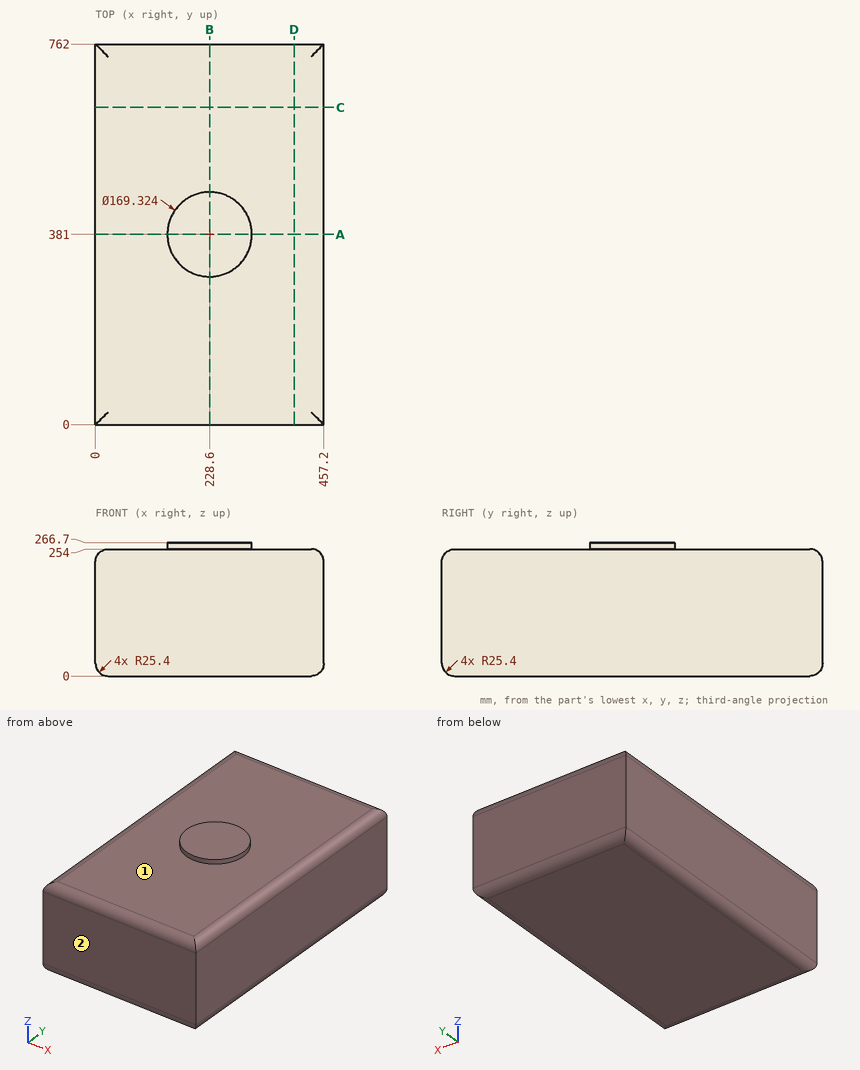
The figure shows three views and two pictorial views of one solid part (mm, origin at its lowest corner). Answer the questions. A direction names the side the tool comes from. Round coordinates to 2 decimals unless told otherwise and drop trailing zeros. Write each loop counter-clockwise with the first axis right and the second up, starting at its lowest first coordinate (ties: lowest second). Pieces come first, ordered by that corner, then holes. Notation, with made-up numbers: M -15.75,36.5 L 40.25,36.5 A37 ccw 40.25,72.5 Z; hole C 21,77 d3. An arc over 180 degrees is marked long. Write each question's results on one line, items separated by ' | '. Start each with the question number.
(1) The part is cut by section B-B, the plane x = 228.6. Write down the section's boundary in (y, z), and give its area (3 significant figures).
(2) Find the intervals of material crossed by line 1 (Z direction, x = 80, y = 39); line 2 (X direction, y = 315.5, z = 14); line 3 (X direction, y = 716, z = 235), in increasing order.
(3) This flat-tipped pin is pushed along its axis until it touches: P1, Ø10, axis at x = 354, y = 638.5, coming from the +Z side. Where does it stop, or does it pass through?
(4) For the marked faces 1 and 2, determine the directions among +Z, -Z, +X, -X, +Y, -Y from which every point of the face is accessible in a straight line to the end or side of a thin tool.
(5) The part is cut by section D-D, the plane x = 397.5. Write down the section's boundary in (y, z), and give its area (3 significant figures).
(6) The part is cut by section C-C, the plane y = 635. Write down the section's boundary in (x, z).
(7) The part is cut by section A-A, the plane y = 381. Write down the section's boundary in (x, z).
Worked answers:
1) outline: M 0,25.4 A25.4 ccw 25.4,0 L 736.6,0 A25.4 ccw 762,25.4 L 762,228.6 A25.4 ccw 736.6,254 L 465.66,254 L 465.66,266.7 L 296.34,266.7 L 296.34,254 L 25.4,254 A25.4 ccw 0,228.6 Z | area: 195,000 mm²
2) line 1: z = 0 to 254 | line 2: x = 2.7 to 454.5 | line 3: x = 0.82 to 456.38
3) P1: stops at z = 254
4) face 1: +Z | face 2: +Z, -Z, +X, -X, -Y
5) outline: M 0,25.4 A25.4 ccw 25.4,0 L 736.6,0 A25.4 ccw 762,25.4 L 762,228.6 A25.4 ccw 736.6,254 L 25.4,254 A25.4 ccw 0,228.6 Z | area: 193,000 mm²
6) outline: M 0,25.4 A25.4 ccw 25.4,0 L 431.8,0 A25.4 ccw 457.2,25.4 L 457.2,228.6 A25.4 ccw 431.8,254 L 25.4,254 A25.4 ccw 0,228.6 Z
7) outline: M 0,25.4 A25.4 ccw 25.4,0 L 431.8,0 A25.4 ccw 457.2,25.4 L 457.2,228.6 A25.4 ccw 431.8,254 L 313.26,254 L 313.26,266.7 L 143.94,266.7 L 143.94,254 L 25.4,254 A25.4 ccw 0,228.6 Z
